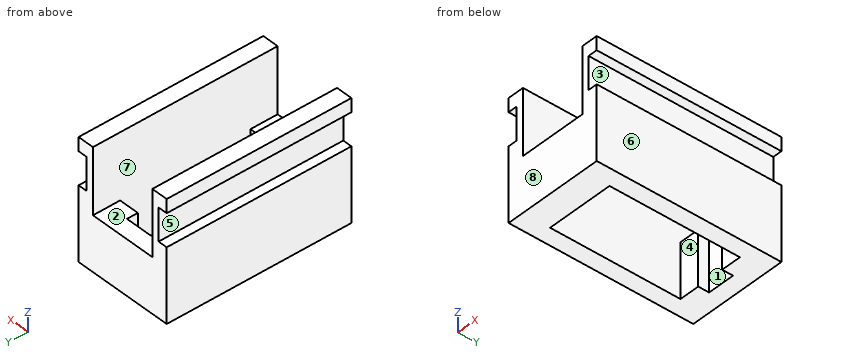
from build123d import *

# Parameters (mm, degrees)
F1_W      = 5
F1_H      = 22
F2_DEPTH  = 6.2
F3_W      = 34
F3_H      = 22
F4_DEPTH  = 3
F6_W      = 12.4
F6_H      = 5
F7_DEPTH  = 12
F8_W      = 5
F8_H      = 2
F9_DEPTH  = 25
F10_W     = 1.7
F10_H     = 6
F11_DEPTH = 34.001


with BuildPart() as f2:
    # F1 (on Right) → F2 (new body, symmetric)
    with BuildSketch(Plane.YZ):
        with Locations((-14.5, 7.65)):
            Rectangle(F1_W, F1_H)
    extrude(amount=F2_DEPTH, both=True)



with BuildPart() as f2b:
    # F1 (on Right) → F2, piece 2 (new body, symmetric)
    with BuildSketch(Plane.YZ):
        with Locations((14.5, 7.65)):
            Rectangle(F1_W, F1_H)
    extrude(amount=F2_DEPTH, both=True)


with BuildPart() as f2_1:
    add(f2.part)

    add(f2b.part)  # F4 merges F2b
    # F3 (on face) → F4 (join)
    with BuildSketch(Plane.YZ.offset(6.2)):
        with Locations((0, 7.65)):
            Rectangle(F3_W, F3_H)
    extrude(amount=F4_DEPTH)

    # F5: F2 across plane


with BuildPart() as f2_2:
    add(f2_1.part)
    add(f2_1.part.mirror(Plane.YZ))

    # F6 (on face) → F7 (cut)
    with BuildSketch(Plane.XY.offset(18.65)):
        with Locations((0, -14.5)):
            Rectangle(F6_W, F6_H)
        with Locations((0, 14.5)):
            Rectangle(F6_W, F6_H)
    extrude(amount=-F7_DEPTH, mode=Mode.SUBTRACT)

    # F8 (on face) → F9 (cut)
    with BuildSketch(Plane.XY.offset(6.65)):
        with Locations((0, 13)):
            Rectangle(F8_W, F8_H)
    extrude(amount=-F9_DEPTH, mode=Mode.SUBTRACT)

    # F10 (on face) → F11 (cut, through all)
    with BuildSketch(Plane.XZ.offset(17)):
        with Locations((-8.35, 13.15)):
            Rectangle(F10_W, F10_H)
        with Locations((8.35, 13.15)):
            Rectangle(F10_W, F10_H)
    extrude(amount=-F11_DEPTH, mode=Mode.SUBTRACT)


solid = f2_2.part
Check sheet for the modelled part. Datum: model origin and axes. Units: mm. Face numbers are marked on the shaded views. A direction names the side the tool comes from. Round coordinates to 2 decimals unless told otherwise and drop trailing zeros. Order: outer loops, then holes, each group sorted by start corner. A loop starts at its lowest first (then second) coordinate and runs counter-clockwise, first axis right, second up.
Q1. Cross-section at B-B, the plane z = 9.5. Enter the section's corners in (x, y), plus the area to 3 significant figures.
Filled sheet:
outline: (-9.2, -17) - (-6.2, -17) - (-6.2, 17) - (-9.2, 17) - close; (6.2, -17) - (9.2, -17) - (9.2, 17) - (6.2, 17) - close
area: 204 mm2
Q2. Cross-section at A-A, the plane x = 1.5. Enter the section's corners in (y, z).
Filled sheet:
outline: (-17, -3.35) - (-12, -3.35) - (-12, 6.65) - (-17, 6.65) - close; (14, -3.35) - (17, -3.35) - (17, 6.65) - (14, 6.65) - close
Q3. Depth check by flat-ended pin: P1, Ø2, axis at x = 3.5, y = 11.5, coming from the -Z side; P2, Ø6, axis at x = 1, y = -7.5, coming from the -Z side; P3, Ø2.5, axis at x = -3, y = 15, coming from the +Z side; P4, Ø3, axis at y = 4, z = 12.5, coming from the -X side. Enter the tip coordinate at first touch or a pass-through.
Filled sheet:
P1: stops at z = -3.35
P2: passes through
P3: stops at z = 6.65
P4: stops at x = -7.5
Q4. Cross-section at D-D, the plane z = 1.25. Enter the section's corners in (x, y).
Filled sheet:
outline: (-9.2, -17) - (9.2, -17) - (9.2, 17) - (-9.2, 17) - close; hole (-6.2, -12) - (6.2, -12) - (6.2, 12) - (2.5, 12) - (2.5, 14) - (-2.5, 14) - (-2.5, 12) - (-6.2, 12) - close
Q5. Draft check along Z on the marked faces 1, 2 and 3. Enter one of: pulls with the +Z half, pulls with the -Z half, needs draft (parallel to the pull), parting line crosses it, or undercut.
Filled sheet:
face 1: needs draft
face 2: pulls with the +Z half
face 3: undercut
Q6. Cross-section at C-C, the plane y = -3.5. Enter the section's corners in (x, z).
Filled sheet:
outline: (-9.2, -3.35) - (-6.2, -3.35) - (-6.2, 18.65) - (-9.2, 18.65) - (-9.2, 16.15) - (-7.5, 16.15) - (-7.5, 10.15) - (-9.2, 10.15) - close; (6.2, -3.35) - (9.2, -3.35) - (9.2, 10.15) - (7.5, 10.15) - (7.5, 16.15) - (9.2, 16.15) - (9.2, 18.65) - (6.2, 18.65) - close
Q7. Set-up check for the marked faces 4, 5, 6, 7 and 8: record each of +Z, -Z, +X, -X, +Y, -Y from which the full face is reachable in a straight line by a thin tool's end or side.
Filled sheet:
face 4: +Z, -Z
face 5: -X, +Y, -Y
face 6: +Z, -Z, +X, +Y, -Y
face 7: +Z
face 8: +Z, -Z, +X, -X, -Y
Q8. Scan lines: L1, parallel to Y at x = -4.75, z = 4.75; L2, parallel to X at y = -1, z = 6; L3, parallel to Y at x = -1.5, z = 3.25. Record each from-to range of solid material in increasing order.
Filled sheet:
L1: y = -17 to -12, 12 to 17
L2: x = -9.2 to -6.2, 6.2 to 9.2
L3: y = -17 to -12, 14 to 17
